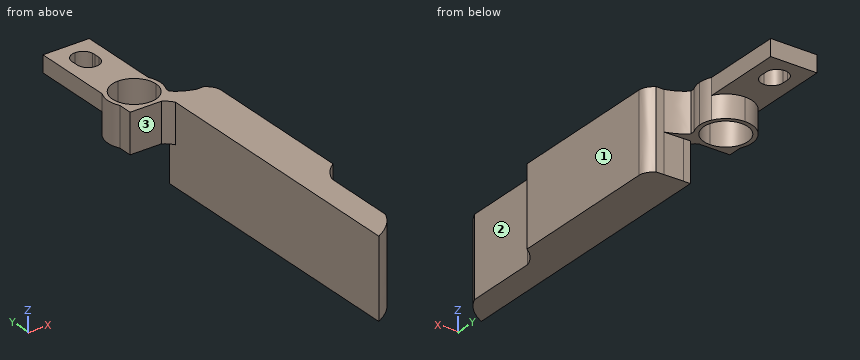
from build123d import *

# Parameters (mm, degrees)
F1_DEPTH = 5.9
F2_DEPTH = 2.5
F3_DEPTH = 11.8


with BuildPart() as f1:
    # F0 (on Top) → F1 (new body)
    with BuildSketch(Plane.XY):
        with BuildLine():
            Line((3.475, 0.65), (3.475, 0))
            ThreePointArc((3.475, 0), (4.7730375063, 0.2208504846), (5.925, 0.8585484677))
            ThreePointArc((5.925, 0.8585484677), (6.5018486959, 1.426237912), (6.95, 2.1001712409))
            Line((6.95, 2.1001712409), (6.95, 5.7498287591))
            ThreePointArc((6.95, 5.7498287591), (5.5051689733, 7.2841723593), (3.475, 7.85))
            Line((3.475, 7.85), (3.475, 7.2))
            ThreePointArc((3.475, 7.2), (5.7907747084, 6.2407747084), (6.75, 3.925))
            ThreePointArc((6.75, 3.925), (5.7907747084, 1.6092252916), (3.475, 0.65))
        make_face()
        with BuildLine():
            Line((0, 5.7498287591), (0, 2.1001712409))
            ThreePointArc((0, 2.1001712409), (0.4481513041, 1.426237912), (1.025, 0.8585484677))
            ThreePointArc((1.025, 0.8585484677), (2.1769624937, 0.2208504846), (3.475, 0))
            Line((3.475, 0), (3.475, 0.65))
            ThreePointArc((3.475, 0.65), (0.2, 3.925), (3.475, 7.2))
            Line((3.475, 7.2), (3.475, 7.85))
            ThreePointArc((3.475, 7.85), (1.4448310267, 7.2841723593), (0, 5.7498287591))
        make_face()
        with BuildLine():
            Line((0, 2.1001712409), (0, 0))
            Line((0, 0), (1.025, 0))
            Line((1.025, 0), (1.025, 0.8585484677))
            ThreePointArc((1.025, 0.8585484677), (0.4481513041, 1.426237912), (0, 2.1001712409))
        make_face()
        with BuildLine():
            Line((1.025, 0.8585484677), (1.025, 0))
            Line((1.025, 0), (3.475, 0))
            ThreePointArc((3.475, 0), (2.1769624937, 0.2208504846), (1.025, 0.8585484677))
        make_face()
        with BuildLine():
            ThreePointArc((0, 5.7498287591), (-0.45, 3.925), (0, 2.1001712409))
            Line((0, 2.1001712409), (0, 5.7498287591))
        make_face()
        with BuildLine():
            Line((6.95, 5.7498287591), (6.95, 2.1001712409))
            ThreePointArc((6.95, 2.1001712409), (7.2858398025, 2.9852526935), (7.4, 3.925))
            ThreePointArc((7.4, 3.925), (7.2858398025, 4.8647473065), (6.95, 5.7498287591))
        make_face()
        with BuildLine():
            ThreePointArc((6.95, 2.1001712409), (6.5018486959, 1.426237912), (5.925, 0.8585484677))
            Line((5.925, 0.8585484677), (5.925, 0))
            Line((5.925, 0), (6.95, 0))
            Line((6.95, 0), (6.95, 1.44))
            Line((6.95, 1.44), (6.95, 1.5))
            Line((6.95, 1.5), (6.95, 2.1001712409))
        make_face()
        with BuildLine():
            ThreePointArc((5.925, 0.8585484677), (4.7730375063, 0.2208504846), (3.475, 0))
            Line((3.475, 0), (4.7, 0))
            Line((4.7, 0), (5.925, 0))
            Line((5.925, 0), (5.925, 0.8585484677))
        make_face()
        with BuildLine():
            Line((5.925, 0), (4.7, 0))
            add(Edge.make_bspline(
                [(4.7, 0), (5.2537494339, -0.3164176305), (5.6369397789, -0.7196032093), (5.925, -1.225)],
                knots=[0, 0, 0, 0, 1.7324116139, 1.7324116139, 1.7324116139, 1.7324116139], degree=3))
            Line((5.925, -1.225), (5.925, -0.079424061))
            Line((5.925, -0.079424061), (5.925, 0))
        make_face()
        with BuildLine():
            Line((6.95, 1.44), (6.95, 0))
            Line((6.95, 0), (9.8284865708, -0.079424061))
            add(Edge.make_bspline(
                [(6.95, 1.5), (7.7566024847, 0.7003984647), (8.7155010551, 0.2800084476), (9.8284865708, -0.079424061)],
                knots=[0, 0, 0, 0, 3.2833314336, 3.2833314336, 3.2833314336, 3.2833314336], degree=3))
            Line((6.95, 1.5), (6.95, 1.44))
        make_face()
    extrude(amount=-F1_DEPTH)

    # F0 (on Top) → F2 (join)
    with BuildSketch(Plane.XY):
        with BuildLine():
            Line((0, 7.85), (0, 5.7498287591))
            ThreePointArc((0, 5.7498287591), (1.4448310267, 7.2841723593), (3.475, 7.85))
            ThreePointArc((3.475, 7.85), (5.5051689733, 7.2841723593), (6.95, 5.7498287591))
            Line((6.95, 5.7498287591), (6.95, 17.9))
            Line((6.95, 17.9), (3.475, 17.9))
            Line((3.475, 17.9), (0, 17.9))
            Line((0, 17.9), (0, 7.85))
        make_face()
        with BuildLine():
            ThreePointArc((1.8276640256, 14.3833613398), (2.3042302705, 15.55900427), (3.475, 16.0474200003))
            ThreePointArc((3.475, 16.0474200003), (4.5253988967, 15.6691157612), (5.0933824344, 14.7079463483))
            Line((5.0933824344, 14.7079463483), (5.1024433757, 14.1442252627))
            Line((5.1024433757, 14.1442252627), (5.113982201, 13.4263440945))
            ThreePointArc((5.113982201, 13.4263440945), (5.1141409801, 13.4131724726), (5.1141939076, 13.4))
            ThreePointArc((5.1141939076, 13.4), (4.6340851277, 12.2409148723), (3.475, 11.7608060924))
            ThreePointArc((3.475, 11.7608060924), (2.2942628451, 12.2629791393), (1.8369719791, 13.4618131819))
            Line((1.8369719791, 13.4618131819), (1.8276640256, 14.3833613398))
        make_face(mode=Mode.SUBTRACT)
    extrude(amount=-F2_DEPTH)

    # F0 (on Top) → F3 (join)
    with BuildSketch(Plane.XY):
        with BuildLine():
            Line((9.8284865708, -25), (5.925, -25))
            Line((5.925, -25), (5.925, -26.9515))
            Line((5.925, -26.9515), (5.925, -28.903))
            Line((5.925, -28.903), (5.925, -43))
            add(Edge.make_bspline(
                [(5.925, -43), (7.9286471009, -41.9465117157), (9.1273570433, -40.6301692128), (9.8284865708, -39.0049032867)],
                knots=[0, 0, 0, 0, 5.5855174476, 5.5855174476, 5.5855174476, 5.5855174476], degree=3))
            Line((9.8284865708, -39.0049032867), (9.8284865708, -28.1095039099))
            Line((9.8284865708, -28.1095039099), (9.8284865708, -25))
        make_face()
        with BuildLine():
            Line((12.1934865708, -25), (9.8284865708, -25))
            Line((9.8284865708, -25), (9.8284865708, -28.1095039099))
            add(Edge.make_bspline(
                [(12.1934865708, -25), (11.0498676077, -25.7655549794), (10.2052474394, -26.863457635), (9.8284865708, -28.1095039099)],
                knots=[0, 0, 0, 0, 3.9066916395, 3.9066916395, 3.9066916395, 3.9066916395], degree=3))
        make_face()
        Polygon((6.95, 0), (5.925, 0), (5.925, -0.079424061), (5.925, -1.225), (5.925, -21.3844068348), (5.925, -22.55), (5.925, -22.9875), (5.925, -25), (9.8284865708, -25), (9.8284865708, -0.079424061), align=None)
        with BuildLine():
            Line((11.0109865708, -0.079424061), (9.8284865708, -0.079424061))
            Line((9.8284865708, -0.079424061), (9.8284865708, -25))
            Line((9.8284865708, -25), (12.1934865708, -25))
            Line((12.1934865708, -25), (12.1934865708, -1.9685707521))
            add(Edge.make_bspline(
                [(11.0109865708, -0.079424061), (11.7086665705, -0.5204698537), (12.1934865708, -1.29045418), (12.1934865708, -1.9685707521)],
                knots=[0, 0, 0, 0, 2.2287174496, 2.2287174496, 2.2287174496, 2.2287174496], degree=3))
        make_face()
    extrude(amount=-F3_DEPTH)


solid = f1.part
Source: CAD feature listing. Evaluate the final solid. Frame: model axes, mm. Face numbers are marked on the shaded views. A direction names the side the tool comes from. Round coordinates to 2 decimals unless told otherwise and drop trailing zeros. Loops run counter-clockwise (first coordinate to the right, second up) from the corner with the lowest first, then second, coordinate; pieces in that order, holes last.
Q1. Ray query, line 1 (X direction, y = -18, z = -9.25) (3 decimals); line 2 (X direction, y = -33, z = -1.75) (3 decimals); line 3 (Y direction, x = 1.5, z = -5.75). Return the intervals inside material, ascending.
Q2. Section A-A, the plane y = 6.5. Return loops of the section in (x, z), plus the area to 3 significant figures.
Q3. Section D-D, the plane y = -38. Return loops of the section in (x, z) (3 decimals), plus the area to 3 significant figures.
Q4. Access query for the marked faces 1, 2 and 3. Directions: +Z, -Z, +X, -X, +Y, -Y. A direction counts if a zero-diameter tool reaches every point of the face in a straight line with its end or side. Return the directions, or none.
Q5. First-contact query: P1, Ø6, axis at x = 7.5, z = -2.5, coming from the +Y side; P2, Ø0.7, axis at y = 2, z = -2, coming from the +X side; P3, Ø3.5, axis at x = 4.5, y = 13, coming from the -Z side; P4, Ø3, axis at y = 10, z = -1, coming from the -X side. Flat tips, straight axial feed; report the tip coordinate or a pass-through.
Q6. Section C-C, the plane y = -9.5. Return loops of the section in (x, z) (3 decimals).
Q7. Section B-B, the plane z = -1.5. State how many separate pieces and enclosed holes the cut face has, plus the area to 3 significant figures.
Solutions:
1. line 1: x = 5.925 to 12.193
1. line 2: x = 5.925 to 9.828
1. line 3: y = 0 to 1.31, 6.54 to 7.32
2. outline: (0, -2.5) - (0.51, -2.5) - (0.51, -5.9) - (1.45, -5.9) - (1.45, 0) - (0, 0) - close; (5.5, -5.9) - (6.44, -5.9) - (6.44, -2.5) - (6.95, -2.5) - (6.95, 0) - (5.5, 0) - close
2. area: 13.6 mm2
3. outline: (5.925, -11.8) - (9.828, -11.8) - (9.828, 0) - (5.925, 0) - close
3. area: 46.1 mm2
4. face 1: +Z, -Z, +X, +Y, -Y
4. face 2: +Z, -Z, +X, -Y
4. face 3: +Z, -Z, -X, -Y
5. P1: stops at y = 17.9
5. P2: stops at x = 7.07
5. P3: stops at z = -2.5
5. P4: stops at x = 0
6. outline: (5.925, -11.8) - (12.193, -11.8) - (12.193, 0) - (5.925, 0) - close
7. separate pieces: 1
7. enclosed holes: 2
7. area: 306 mm2
